```python
from build123d import *

# Parameters (mm, degrees)
BOSS_EXTRUDE1_DEPTH = 152.4
CUT_EXTRUDE1_DEPTH  = 239.273120599
CUT_EXTRUDE2_DEPTH  = 218.110576665


with BuildPart() as part:
    # Sketch2 → Boss-Extrude1 (new, symmetric)
    with BuildSketch(Plane.XY):
        with BuildLine():
            Line((-50.8, 0), (50.8, 0))
            Line((50.8, 0), (50.8, 152.4))
            Line((50.8, 152.4), (47.625, 152.4))
            ThreePointArc((47.625, 152.4), (45.37993597, 151.47006403), (44.45, 149.225))
            Line((44.45, 149.225), (44.45, 9.525))
            ThreePointArc((44.45, 9.525), (43.52006403, 7.27993597), (41.275, 6.35))
            Line((41.275, 6.35), (-47.625, 6.35))
            ThreePointArc((-47.625, 6.35), (-49.87006403, 5.42006403), (-50.8, 3.175))
            Line((-50.8, 3.175), (-50.8, 0))
        make_face()
    extrude(amount=BOSS_EXTRUDE1_DEPTH, both=True)

    # SurfaceCut1
    split(bisect_by=Plane(origin=(0, 0, -38.1), x_dir=(-1, 0, 0), z_dir=(0, 0, -1)), keep=Keep.TOP)

    # Sketch3 → Cut-Extrude1 (cut, through all)
    with BuildSketch(Plane(origin=(50.8, 0, 0), x_dir=(0, 0, -1), z_dir=(1, 0, 0))):
        with BuildLine():
            Line((145.961940777, 144.386940777), (145.961940777, 106.286940777))
            ThreePointArc((145.961940777, 106.286940777), (141.211940777, 101.536940777), (136.461940777, 106.286940777))
            Line((136.461940777, 106.286940777), (136.461940777, 144.386940777))
            ThreePointArc((136.461940777, 144.386940777), (141.211940777, 149.136940777), (145.961940777, 144.386940777))
        make_face()
        with BuildLine():
            Line((145.961940777, 52.463059223), (145.961940777, 14.363059223))
            ThreePointArc((145.961940777, 14.363059223), (141.211940777, 9.613059223), (136.461940777, 14.363059223))
            Line((136.461940777, 14.363059223), (136.461940777, 52.463059223))
            ThreePointArc((136.461940777, 52.463059223), (141.211940777, 57.213059223), (145.961940777, 52.463059223))
        make_face()
        with BuildLine():
            Line((44.538059223, 52.463059223), (44.538059223, 14.363059223))
            ThreePointArc((44.538059223, 14.363059223), (49.288059223, 9.613059223), (54.038059223, 14.363059223))
            Line((54.038059223, 14.363059223), (54.038059223, 52.463059223))
            ThreePointArc((54.038059223, 52.463059223), (49.288059223, 57.213059223), (44.538059223, 52.463059223))
        make_face()
        with BuildLine():
            Line((44.538059223, 144.386940777), (44.538059223, 106.286940777))
            ThreePointArc((44.538059223, 106.286940777), (49.288059223, 101.536940777), (54.038059223, 106.286940777))
            Line((54.038059223, 106.286940777), (54.038059223, 144.386940777))
            ThreePointArc((54.038059223, 144.386940777), (49.288059223, 149.136940777), (44.538059223, 144.386940777))
        make_face()
        with BuildLine():
            Line((107.95, 98.425), (107.95, 60.325))
            ThreePointArc((107.95, 60.325), (95.25, 47.625), (82.55, 60.325))
            Line((82.55, 60.325), (82.55, 98.425))
            ThreePointArc((82.55, 98.425), (95.25, 111.125), (107.95, 98.425))
        make_face()
    extrude(amount=-CUT_EXTRUDE1_DEPTH, mode=Mode.SUBTRACT)

    # Sketch4 → Cut-Extrude2 (cut, through all)
    with BuildSketch(Plane(origin=(0, 6.35, 0), x_dir=(1, 0, 0), z_dir=(0, 1, 0))):
        with BuildLine():
            Line((-42.8625, 98.5139), (-17.4625, 98.5139))
            ThreePointArc((-17.4625, 98.5139), (-14.1986, 95.25), (-17.4625, 91.9861))
            Line((-17.4625, 91.9861), (-42.8625, 91.9861))
            ThreePointArc((-42.8625, 91.9861), (-46.1264, 95.25), (-42.8625, 98.5139))
        make_face()
        with BuildLine():
            Line((7.9375, 98.5139), (33.3375, 98.5139))
            ThreePointArc((33.3375, 98.5139), (36.6014, 95.25), (33.3375, 91.9861))
            Line((33.3375, 91.9861), (7.9375, 91.9861))
            ThreePointArc((7.9375, 91.9861), (4.6736, 95.25), (7.9375, 98.5139))
        make_face()
        with BuildLine():
            Line((-17.4625, 142.507990512), (7.9375, 142.507990512))
            ThreePointArc((7.9375, 142.507990512), (11.2014, 139.244090512), (7.9375, 135.980190512))
            Line((7.9375, 135.980190512), (-17.4625, 135.980190512))
            ThreePointArc((-17.4625, 135.980190512), (-20.7264, 139.244090512), (-17.4625, 142.507990512))
        make_face()
        with BuildLine():
            Line((-17.4625, 47.992009488), (7.9375, 47.992009488))
            ThreePointArc((7.9375, 47.992009488), (11.2014, 51.255909488), (7.9375, 54.519809488))
            Line((7.9375, 54.519809488), (-17.4625, 54.519809488))
            ThreePointArc((-17.4625, 54.519809488), (-20.7264, 51.255909488), (-17.4625, 47.992009488))
        make_face()
    extrude(amount=-CUT_EXTRUDE2_DEPTH, mode=Mode.SUBTRACT)


solid = part.part
```
CAD build for the part. Positions are in the model's coordinates, mm. A direction names the side the tool comes from. Round coordinates to 2 decimals unless told otherwise and drop trailing zeros. Order: outer loops, then holes, each group sorted by start corner. A loop starts at its lowest first (then second) coordinate and runs counter-clockwise, first axis right, second up. Notation, with made-up numbers: (-26, -28.5) - (16, -28.5) arc R13 ccw to (16, -18.5) - close; hole circle Ø9 at (11.25, -14.5). An arc over 180 degrees is marked (long way). Use CSV: the item, a comma, the result in double quotes. Start each with the question number.
1) Saw through at D-D (y = 96). List the corners of the cut face in (x, z).
2) Tool access for faces 1 (the cylindrical face through (36.6, 3.2, -95.3)), 2 (the cylindrical face through (47.67, 47.63, -95.53)): list every direction of +Z, -Z, +X, -X, +Y, -Y with a clear straight run to the whole face (end or side of a thin tool).
3) Saw through at C-C (z = -87). List the corners of the cut face in (x, y) (3 decimals).
4) Two-plate mould, pull along Z, no slides. Class faces 3 (the flat face through (45, 54, -152.4)), 4 (the flat face through (48, 126, -44.538)), 5 (the flat face through (20, 3, -98.514)), 6 (the flat face through (-3, 6.35, -94)): pulls with the +Z half, pulls with the -Z half, needs draft (parallel to the pull), parting line crosses it, or undercut.
5) Saw through at B-B (x = 21). List the corners of the cut face in (y, z).
6) Pin check, flat tip, straight feed: pin 1 Ø5 at (x, z) = (2.5, -99.5) entering from +Y. Stop position of the tip, or through.
7) Saw through at A-A (y = 115). List the corners of the cut face in (x, z), and give its area (3 significant figures).
8) Wall check: L1, parallel to Z at x = 44.5, y = 40.5; L2, parallel to X at y = 48, z = -133; L3, parallel to Y at x = 38.5, z = -103.5. Give the ranges that are in metal, low to high. Write a range as [from, to].
Values follow:
1,outline,"(44.45, -152.4) - (50.8, -152.4) - (50.8, -107.95) - (44.45, -107.95) - close; (44.45, -82.55) - (50.8, -82.55) - (50.8, -38.1) - (44.45, -38.1) - close"
2,face 1,"+Y, -Y"
2,face 2,"+X, -X"
3,outline,"(-50.8, 0) - (50.8, 0) - (50.8, 50.67) - (44.45, 50.67) - (44.45, 9.525) arc R3.175 cw to (41.275, 6.35) - (-47.625, 6.35) arc R3.175 ccw to (-50.8, 3.175) - close; (44.45, 108.08) - (50.8, 108.08) - (50.8, 152.4) - (47.625, 152.4) arc R3.175 ccw to (44.45, 149.225) - close"
4,face 3,"pulls with the -Z half"
4,face 4,"undercut"
4,face 5,"undercut"
4,face 6,"needs draft"
5,outline,"(0, -152.4) - (6.35, -152.4) - (6.35, -98.51) - (0, -98.51) - close; (0, -91.99) - (6.35, -91.99) - (6.35, -38.1) - (0, -38.1) - close"
6,pin 1,"stops at y = 6.35"
7,outline,"(44.45, -152.4) - (50.8, -152.4) - (50.8, -145.96) - (44.45, -145.96) - close; (44.45, -136.46) - (50.8, -136.46) - (50.8, -54.04) - (44.45, -54.04) - close; (44.45, -44.54) - (50.8, -44.54) - (50.8, -38.1) - (44.45, -38.1) - close"
7,area,"605 mm2"
8,L1,"z = [-152.4, -145.96], [-136.46, -54.04], [-44.54, -38.1]"
8,L2,"x = [44.45, 50.8]"
8,L3,"y = [0, 6.35]"
